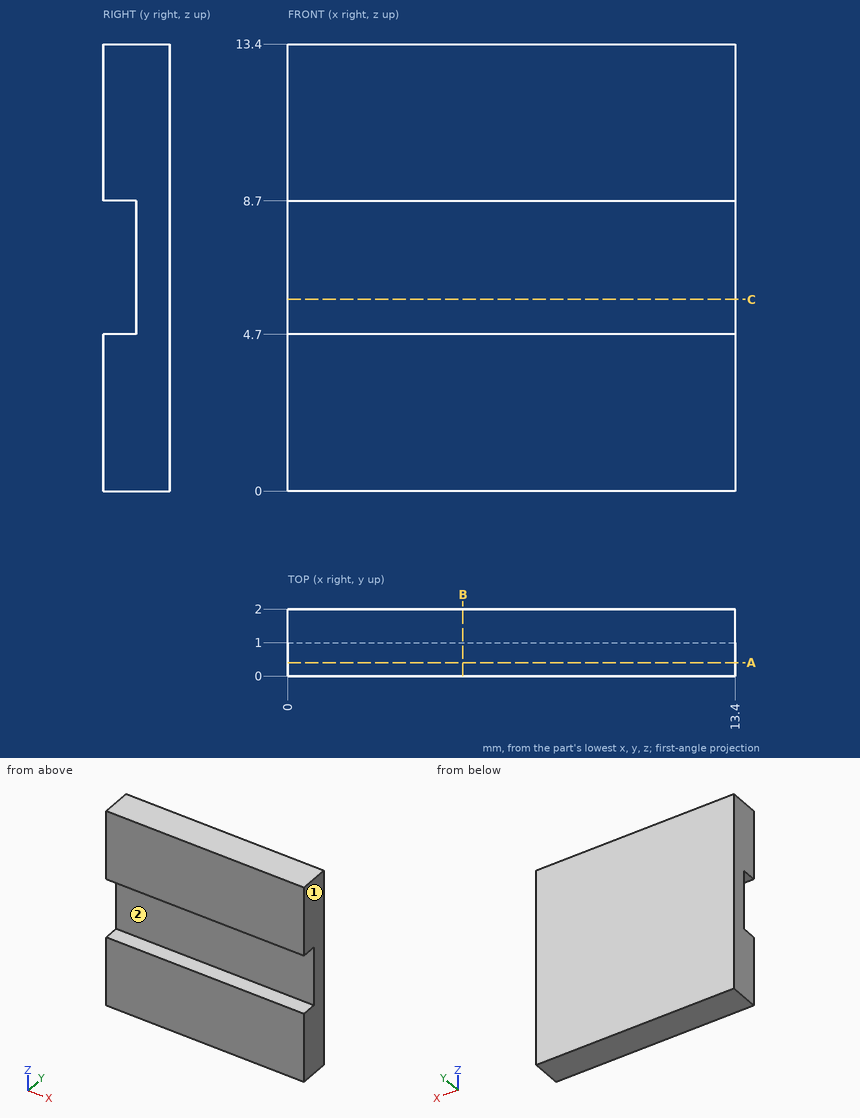
Design review of the part shown in the three views and the two pictorial views. Dimensions are in mm from the part's minimum x, y and z. A direction names the side the tool comes from. Round coordinates to 2 decimals unless told otherwise and drop trailing zeros. Write each loop counter-clockwise with the first axis right and the second up, starting at its lowest first coordinate (ties: lowest second). Pieces come first, ordered by that corner, then holes. Notation, with made-up numbers: (33, 55) -> (66, 55) arc R18 cw to (66, 81) -> close; hole circle Ø4 at (-15, 58.5). An arc over 180 degrees is marked (long way). One line per question, with ' | ' between items. Start each with the question number.
1) Add section A-A (y = 0.4). Write out the cut boundary in (x, z).
2) Wall thickness on line 1 along Z through (x, y) = (12.75, 0.55); line 2 along Y through (x, z) = (12.75, 6): over which ranges is each line inside the solid? List them lowest first.
3) Machinability: for the marked faces 1 and 2, which of the approach directions +Z, -Z, +X, -X, +Y, -Y give a long, thin tool a straight path to every point of the face, cutting with its end or side? Answer none if there is none.
4) Add section C-C (z = 5.75). Write out the cut boundary in (x, y), and give its area (3 significant figures).
5) Add section B-B (x = 5.25). Write out the cut boundary in (y, z), and give its area (3 significant figures).
Reported:
1) outline: (0, 0) -> (13.4, 0) -> (13.4, 4.7) -> (0, 4.7) -> close; (0, 8.7) -> (13.4, 8.7) -> (13.4, 13.4) -> (0, 13.4) -> close
2) line 1: z = 0 to 4.7, 8.7 to 13.4 | line 2: y = 1 to 2
3) face 1: +Z, -Z, +X, +Y, -Y | face 2: +X, -X, -Y
4) outline: (0, 1) -> (13.4, 1) -> (13.4, 2) -> (0, 2) -> close | area: 13.4 mm²
5) outline: (0, 0) -> (2, 0) -> (2, 13.4) -> (0, 13.4) -> (0, 8.7) -> (1, 8.7) -> (1, 4.7) -> (0, 4.7) -> close | area: 22.8 mm²
